from build123d import *

# Parameters (mm, degrees)
PAD_DEPTH       = 3
PAD001_DEPTH    = 10
SKETCH002_R     = 5
PAD002_DEPTH    = 3
POCKET_DEPTH    = 3
SKETCH004_R     = 1.7
POCKET001_DEPTH = 3
SKETCH005_R     = 5
PAD003_DEPTH    = 3
SKETCH006_R     = 1.7
POCKET002_DEPTH = 2.8
POCKET003_DEPTH = 3
SKETCH008_R     = 4
POCKET004_DEPTH = 3
POCKET005_DEPTH = 3
SKETCH010_R     = 1.7
POCKET006_DEPTH = 3
POCKET007_DEPTH = 3
SKETCH012_R     = 1.7
POCKET008_DEPTH = 3
POCKET009_DEPTH = 3
SKETCH014_R     = 1.7
POCKET010_DEPTH = 3
POCKET011_DEPTH = 3
SKETCH016_R     = 1.7
POCKET012_DEPTH = 3


with BuildPart() as part:
    # Sketch → Pad (new body)
    with BuildSketch(Plane.XY):
        with BuildLine():
            ThreePointArc((0, 10), (2.928932, 2.928932), (10, 0))
            Line((110, 0), (10, 0))
            ThreePointArc((110, 0), (117.071068, 2.928932), (120, 10))
            Line((120, 44), (120, 10))
            ThreePointArc((120, 44), (117.071068, 51.071068), (110, 54))
            Line((10, 54), (110, 54))
            ThreePointArc((10, 54), (2.928932, 51.071068), (0, 44))
            Line((0, 10), (0, 44))
        make_face()
    extrude(amount=PAD_DEPTH)

    # Sketch001 → Pad001 (new body)
    with BuildSketch(Plane.XY.offset(3)):
        with BuildLine():
            ThreePointArc((0, 10), (2.928932, 2.928932), (10, 0))
            Line((110, 0), (10, 0))
            ThreePointArc((110, 0), (117.071068, 2.928932), (120, 10))
            Line((120, 44), (120, 10))
            ThreePointArc((120, 44), (117.071068, 51.071068), (110, 54))
            Line((10, 54), (110, 54))
            ThreePointArc((10, 54), (2.928932, 51.071068), (0, 44))
            Line((0, 10), (0, 44))
        make_face()
        with BuildLine():
            ThreePointArc((10, 52), (4.343146, 49.656854), (2, 44))
            Line((2, 44), (2, 31))
            Line((2, 31), (5, 31))
            Line((5, 31), (5, 23))
            Line((5, 23), (2, 23))
            Line((2, 23), (2, 10))
            ThreePointArc((2, 10), (4.343146, 4.343146), (10, 2))
            Line((10, 2), (27, 2))
            Line((27, 2), (27, 5))
            Line((27, 5), (35, 5))
            Line((35, 5), (35, 2))
            Line((35, 2), (85, 2))
            Line((85, 2), (85, 5))
            Line((85, 5), (93, 5))
            Line((93, 5), (93, 2))
            Line((93, 2), (110, 2))
            ThreePointArc((110, 2), (115.656854, 4.343146), (118, 10))
            Line((118, 23), (118, 10))
            Line((115, 23), (118, 23))
            Line((115, 31), (115, 23))
            Line((118, 31), (115, 31))
            Line((118, 44), (118, 31))
            ThreePointArc((118, 44), (115.656854, 49.656854), (110, 52))
            Line((93, 52), (110, 52))
            Line((93, 49), (93, 52))
            Line((85, 49), (93, 49))
            Line((85, 52), (85, 49))
            Line((35, 52), (85, 52))
            Line((35, 49), (35, 52))
            Line((27, 49), (35, 49))
            Line((27, 52), (27, 49))
            Line((10, 52), (27, 52))
        make_face(mode=Mode.SUBTRACT)
    extrude(amount=PAD001_DEPTH)

    # Sketch002 → Pad002 (new body)
    with BuildSketch(Plane.XY.offset(3)):
        with Locations((8, 45)):
            Circle(SKETCH002_R)
        with Locations((22, 45)):
            Circle(SKETCH002_R)
        with Locations((8, 9)):
            Circle(SKETCH002_R)
        with Locations((22, 9)):
            Circle(SKETCH002_R)
        with Locations((98, 45)):
            Circle(SKETCH002_R)
        with Locations((112, 45)):
            Circle(SKETCH002_R)
        with Locations((98, 9)):
            Circle(SKETCH002_R)
        with Locations((112, 9)):
            Circle(SKETCH002_R)
    extrude(amount=PAD002_DEPTH)

    # Sketch003 → Pocket (cut)
    with BuildSketch(Plane.XY.offset(6)):
        Polygon((10.857884, 43.35), (10.857884, 46.65), (8, 48.3), (5.142116, 46.65), (5.142116, 43.35), (8, 41.7), align=None)
        Polygon((24.857884, 43.35), (24.857884, 46.65), (22, 48.3), (19.142116, 46.65), (19.142116, 43.35), (22, 41.7), align=None)
        Polygon((10.857884, 7.35), (10.857884, 10.65), (8, 12.3), (5.142116, 10.65), (5.142116, 7.35), (8, 5.7), align=None)
        Polygon((22, 5.7), (24.857884, 7.35), (24.857884, 10.65), (22, 12.3), (19.142116, 10.65), (19.142116, 7.35), align=None)
        Polygon((95.142116, 46.65), (95.142116, 43.35), (98, 41.7), (100.857884, 43.35), (100.857884, 46.65), (98, 48.3), align=None)
        Polygon((109.142116, 43.35), (112, 41.7), (114.857884, 43.35), (114.857884, 46.65), (112, 48.3), (109.142116, 46.65), align=None)
        Polygon((112, 5.7), (114.857884, 7.35), (114.857884, 10.65), (112, 12.3), (109.142116, 10.65), (109.142116, 7.35), align=None)
        Polygon((95.142116, 7.35), (98, 5.7), (100.857884, 7.35), (100.857884, 10.65), (98, 12.3), (95.142116, 10.65), align=None)
    extrude(amount=-POCKET_DEPTH, mode=Mode.SUBTRACT)

    # Sketch004 → Pocket001 (cut)
    with BuildSketch(Plane.XY.offset(3)):
        with Locations((8, 45)):
            Circle(SKETCH004_R)
        with Locations((22, 45)):
            Circle(SKETCH004_R)
        with Locations((8, 9)):
            Circle(SKETCH004_R)
        with Locations((22, 9)):
            Circle(SKETCH004_R)
        with Locations((98, 45)):
            Circle(SKETCH004_R)
        with Locations((112, 45)):
            Circle(SKETCH004_R)
        with Locations((98, 9)):
            Circle(SKETCH004_R)
        with Locations((112, 9)):
            Circle(SKETCH004_R)
    extrude(amount=-POCKET001_DEPTH, mode=Mode.SUBTRACT)

    # Sketch005 → Pad003 (new body)
    with BuildSketch(Plane.XY.offset(3)):
        with Locations((41.5, 45.5)):
            Circle(SKETCH005_R)
        with Locations((78.5, 45.5)):
            Circle(SKETCH005_R)
        with Locations((78.5, 8.5)):
            Circle(SKETCH005_R)
        with Locations((41.5, 8.5)):
            Circle(SKETCH005_R)
    extrude(amount=PAD003_DEPTH)

    # Sketch006 → Pocket002 (cut)
    with BuildSketch(Plane.XY.offset(6)):
        with Locations((41.5, 45.5)):
            Circle(SKETCH006_R)
        with Locations((78.5, 45.5)):
            Circle(SKETCH006_R)
        with Locations((78.5, 8.5)):
            Circle(SKETCH006_R)
        with Locations((41.5, 8.5)):
            Circle(SKETCH006_R)
    extrude(amount=-POCKET002_DEPTH, mode=Mode.SUBTRACT)

    # Sketch007 → Pocket003 (cut)
    with BuildSketch(Plane(origin=(0, 0, 0), x_dir=(1, 0, 0), z_dir=(0, 0, -1))):
        Polygon((44.357884, -10.15), (44.357884, -6.85), (41.5, -5.2), (38.642116, -6.85), (38.642116, -10.15), (41.5, -11.8), align=None)
        Polygon((81.357884, -10.15), (81.357884, -6.85), (78.5, -5.2), (75.642116, -6.85), (75.642116, -10.15), (78.5, -11.8), align=None)
        Polygon((81.357884, -43.85), (78.5, -42.2), (75.642116, -43.85), (75.642116, -47.15), (78.5, -48.8), (81.357884, -47.15), align=None)
        Polygon((44.357884, -43.85), (41.5, -42.2), (38.642116, -43.85), (38.642116, -47.15), (41.5, -48.8), (44.357884, -47.15), align=None)
    extrude(amount=-POCKET003_DEPTH, mode=Mode.SUBTRACT)

    # Sketch008 → Pocket004 (cut)
    with BuildSketch(Plane.XY.offset(3)):
        with Locations((60, 27)):
            Circle(SKETCH008_R)
    extrude(amount=-POCKET004_DEPTH, mode=Mode.SUBTRACT)

    # Sketch009 → Pocket005 (cut)
    with BuildSketch(Plane(origin=(0, 31, 0), x_dir=(-1, 0, 0), z_dir=(0, 1, 0))):
        Polygon((33.598076, 9.5), (31, 11), (28.401924, 9.5), (28.401924, 6.5), (31, 5), (33.598076, 6.5), align=None)
        Polygon((91.598076, 9.5), (89, 11), (86.401924, 9.5), (86.401924, 6.5), (89, 5), (91.598076, 6.5), align=None)
    extrude(amount=-POCKET005_DEPTH, mode=Mode.SUBTRACT)

    # Sketch010 → Pocket006 (cut)
    with BuildSketch(Plane.XZ.offset(-52)):
        with Locations((31, 8)):
            Circle(SKETCH010_R)
        with Locations((89, 8)):
            Circle(SKETCH010_R)
    extrude(amount=-POCKET006_DEPTH, mode=Mode.SUBTRACT)

    # Sketch011 → Pocket007 (cut)
    with BuildSketch(Plane(origin=(0, 5, 0), x_dir=(-1, 0, 0), z_dir=(0, 1, 0))):
        Polygon((-86.401924, 9.5), (-89, 11), (-91.598076, 9.5), (-91.598076, 6.5), (-89, 5), (-86.401924, 6.5), align=None)
        Polygon((-28.401924, 9.5), (-31, 11), (-33.598076, 9.5), (-33.598076, 6.5), (-31, 5), (-28.401924, 6.5), align=None)
    extrude(amount=-POCKET007_DEPTH, mode=Mode.SUBTRACT)

    # Sketch012 → Pocket008 (cut)
    with BuildSketch(Plane(origin=(0, 2, 0), x_dir=(-1, 0, 0), z_dir=(0, 1, 0))):
        with Locations((-89, 8)):
            Circle(SKETCH012_R)
        with Locations((-31, 8)):
            Circle(SKETCH012_R)
    extrude(amount=-POCKET008_DEPTH, mode=Mode.SUBTRACT)

    # Sketch013 → Pocket009 (cut)
    with BuildSketch(Plane(origin=(115, 0, 0), x_dir=(0, -1, 0), z_dir=(-1, 0, 0))):
        Polygon((-24.401924, 6.5), (-24.401924, 9.5), (-27, 11), (-29.598076, 9.5), (-29.598076, 6.5), (-27, 5), align=None)
    extrude(amount=-POCKET009_DEPTH, mode=Mode.SUBTRACT)

    # Sketch014 → Pocket010 (cut)
    with BuildSketch(Plane(origin=(118, 0, 0), x_dir=(0, -1, 0), z_dir=(-1, 0, 0))):
        with Locations((-27, 8)):
            Circle(SKETCH014_R)
    extrude(amount=-POCKET010_DEPTH, mode=Mode.SUBTRACT)

    # Sketch015 → Pocket011 (cut)
    with BuildSketch(Plane(origin=(85, 0, 0), x_dir=(0, -1, 0), z_dir=(-1, 0, 0))):
        Polygon((29.598076, 6.5), (29.598076, 9.5), (27, 11), (24.401924, 9.5), (24.401924, 6.5), (27, 5), align=None)
    extrude(amount=-POCKET011_DEPTH, mode=Mode.SUBTRACT)

    # Sketch016 → Pocket012 (cut)
    with BuildSketch(Plane.YZ.offset(2)):
        with Locations((27, 8)):
            Circle(SKETCH016_R)
    extrude(amount=-POCKET012_DEPTH, mode=Mode.SUBTRACT)


solid = part.part
Design review of the part built by this model. Coordinates are the model's own, in mm. A direction names the side the tool comes from. Round coordinates to 2 decimals unless told otherwise and drop trailing zeros. Write each loop counter-clockwise with the first axis right and the second up, starting at its lowest first coordinate (ties: lowest second). Pieces come first, ordered by that corner, then holes. Notation, with made-up numbers: (-5, 59) -> (29, 59) arc R17 ccw to (29, 76) -> close; hole circle Ø8 at (-20.5, 58.25). An arc over 180 degrees is marked (long way). One line per item, written item: value. Start each with the question number.
Q1. Add section B-B (x = 15). Give the boundary of the cut face in (y, z), then the cut area to 3 significant figures.
Q2. Add section A-A (x = 60). Give the boundary of the cut face in (y, z).
Q3. Insertion check: P1, Ø3.5, axis at y = 3.5, z = 8.5, coming from the -X side; P2, Ø2.5, axis at x = 30, z = 8.5, coming from the +Y side; P3, Ø3.5, axis at y = 50.5, z = 9.5, coming from the +X side; P4, Ø1.7, axis at y = 27, z = 8, coming from the -X side. Each pin has a flat end and moves straight along its axis. Give the tip position at first contact, or say it passes through.
Q4. Tool access review of faces 1 (the face through (44.358, 46, 1)), 2 (the face through (32.62, 52.99, 8.51)), 3 (the face through (115.3, 9.1, 6)): name each direction out of +Z, -Z, +X, -X, +Y, -Y from which nothing blocks a thin tool from reaching the whole face with its end or side.
Q5. To check wall thickness, follow probe 1 along X at (y, z) = (21, 8.75); probe 2 along Y at (x, z) = (49, 4.25); probe 3 along Y at (x, z) = (112, 1.75). State the ranges of each line that lie inside material, in increasing order.
Response:
1. outline: (0, 0) -> (54, 0) -> (54, 13) -> (52, 13) -> (52, 3) -> (2, 3) -> (2, 13) -> (0, 13) -> close
1. area: 202 mm^2
2. outline: (0, 0) -> (23, 0) -> (23, 3) -> (2, 3) -> (2, 13) -> (0, 13) -> close; (31, 0) -> (54, 0) -> (54, 13) -> (52, 13) -> (52, 3) -> (31, 3) -> close
3. P1: stops at x = 1.2
3. P2: stops at y = 54
3. P3: stops at x = 118.8
3. P4: stops at x = 2
4. face 1: -Z
4. face 2: +Y
4. face 3: +Z
5. probe 1: x = 0 to 2, 118 to 120
5. probe 2: y = 0 to 2, 52 to 54
5. probe 3: y = 0.2 to 7.3, 10.7 to 43.3, 46.7 to 53.8
